from build123d import *

# Parameters (mm, degrees)
SKETCH7_R          = 2.3876
CUT_EXTRUDE3_DEPTH = 12.7


with BuildPart() as part:
    # Sketch1 → Revolve-Thin1 (revolve)
    with BuildSketch(Plane(origin=(0, 0, 0), x_dir=(0, 0, -1), z_dir=(1, 0, 0)), mode=Mode.PRIVATE) as revolve_thin1_sk:
        with BuildLine():
            ThreePointArc((0, 0), (13.92977193, 42.243362599), (50.254629325, 67.915233681))
            Line((50.254629325, 67.915233681), (77.352878934, 76.2))
            Line((77.352878934, 76.2), (90.052878934, 78.668629926))
            Line((90.052878934, 78.668629926), (103.700637121, 81.321485381))
            ThreePointArc((103.700637121, 81.321485381), (107.388816105, 83.515721298), (108.839, 87.554817996))
            Line((108.839, 87.554817996), (108.839, 114.3))
            Line((108.839, 114.3), (106.299, 114.3))
            Line((106.299, 114.3), (106.299, 87.554817996))
            ThreePointArc((106.299, 87.554817996), (105.428889663, 85.131359977), (103.215982272, 83.814818427))
            Line((103.215982272, 83.814818427), (89.568224085, 81.161962972))
            Line((89.568224085, 81.161962972), (76.737554038, 78.667933362))
            Line((76.737554038, 78.667933362), (49.512005195, 70.344247761))
            ThreePointArc((49.512005195, 70.344247761), (11.887975504, 43.754212477), (-2.54, 0))
            Line((-2.54, 0), (0, 0))
        make_face()
    revolve(revolve_thin1_sk.sketch.rotate(Axis((0, 0, -134.341700673), (0, 0, 1)), 90), axis=Axis((0, 0, -134.341700673), (0, 0, 1)))

    # Sketch5 → Cut-Revolve1 (revolve, cut)
    with BuildSketch(Plane(origin=(0, 0, 0), x_dir=(0, 0, -1), z_dir=(1, 0, 0)), mode=Mode.PRIVATE) as cut_revolve1_sk:
        with BuildLine():
            Line((-1.27, 0), (-23.88640598, 0))
            Line((-23.88640598, 0), (-23.88640598, 127.217845703))
            Line((-23.88640598, 127.217845703), (116.900257224, 127.217845703))
            Line((116.900257224, 127.217845703), (116.900257224, 70.000934593))
            Line((116.900257224, 70.000934593), (90.052878934, 70.000934593))
            Line((90.052878934, 70.000934593), (90.052878934, 79.962400129))
            Line((90.052878934, 79.962400129), (77.045216486, 77.433966681))
            Line((77.045216486, 77.433966681), (49.88331726, 69.129740721))
            ThreePointArc((49.88331726, 69.129740721), (12.908873717, 42.998787538), (-1.27, 0))
        make_face()
    revolve(cut_revolve1_sk.sketch.rotate(Axis((0, 0, -134.341700673), (0, 0, 1)), 90), axis=Axis((0, 0, -134.341700673), (0, 0, 1)), mode=Mode.SUBTRACT)

    # Sketch7 → Cut-Extrude3 (cut, symmetric)
    with BuildSketch(Plane.XY):
        with Locations(Location((0, 0, 0), (0, 0, 90))):
            Circle(SKETCH7_R)
    extrude(amount=CUT_EXTRUDE3_DEPTH, both=True, mode=Mode.SUBTRACT)


solid = part.part
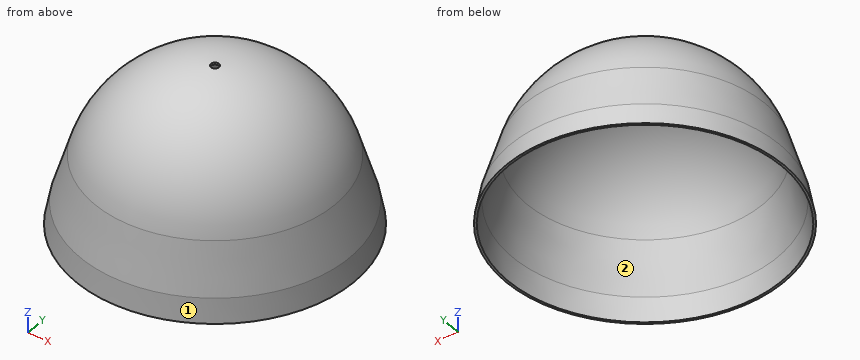
Part model, mm, in its own coordinate system. Face numbers are marked on the shaded views. Coordinates: 2 decimals unless noted, no trailing zeros. Loops run counter-clockwise (first coordinate to the right, second up) from the corner with the lowest first, then second, coordinate; pieces in that order, holes last. Notation, with made-up numbers: (-5, 44) - (3, 44) arc R26 ccw to (3, 68) - close; hole circle Ø4 at (67.25, 64). An arc over 180 degrees is marked (long way). Write each question's results on one line, items separated by ' | '. Start each with the question number.
Q1. Slice it at C-C on z = -73.5. Give the cut face in (x, y).
Q2. Slice it at A-A on y = 0. Give the cut face in (x, z), and give its area (3 significant figures).
Q3. Probe line 1 along Y through (x, z) = (27, -74); line 2 along Y through (x, z) = (17.5, -31); line 3 along X through (y, z) = (-32, -35). List the from-to ranges inside material, lowest first.
Q4. Two-plate mould, pull along X, no slides. Class the marked faces 1 and 2: +X half, -X half, draft (parallel to the pull), parting line (faces both ways), or undercut.
Q5. Drop flat-ended pins along their axis: pin 1 Ø3 at (x, z) = (24.5, -65) entering from +Y; pin 2 Ø6 at (y, z) = (-50.5, -57.5) entering from -X; pin 3 Ø1 at (x, z) = (-6, -51) entering from +Y. Give the stop position or say it passes through.
Answer:
1) outline: circle Ø152.7 at (0, 0); hole circle Ø150.04 at (0, 0)
2) outline: (-79.96, -90.05) - (-78.67, -90.05) - (-76.2, -77.35) - (-67.92, -50.25) arc R71.02 cw to (-2.39, -0.04) - (-2.39, 1.23) arc R72.29 ccw to (-69.13, -49.88) - (-77.43, -77.05) - close; (2.39, -0.04) arc R71.02 cw to (67.92, -50.25) - (76.2, -77.35) - (78.67, -90.05) - (79.96, -90.05) - (77.43, -77.05) - (69.13, -49.88) arc R72.29 ccw to (2.39, 1.23) - close | area: 331 mm2
3) line 1: y = -71.58 to -70.16, 70.16 to 71.58 | line 2: y = -57.6 to -56, 56 to 57.6 | line 3: x = -53.89 to -52.18, 52.18 to 53.89
4) face 1: parting line | face 2: undercut
5) pin 1: stops at y = 70.27 | pin 2: stops at x = -53.65 | pin 3: stops at y = 69.37
